```python
from build123d import *

# Parameters (mm, degrees)
F0_W     = 12.7
F0_H     = 21.59
F0_W_2   = 21.59
F0_H_2   = 12.7
F1_DEPTH = 50.8
F2_R     = 4.7625
F3_DEPTH = 12.7
F4_R     = 4.7625
F5_DEPTH = 12.7


with BuildPart() as f1:
    # F0 (on Top) → F1 (new body)
    with BuildSketch(Plane.XY):
        Polygon((34.29, 0), (0, 0), (0, -34.29), (12.7, -34.29), (12.7, -12.7), (34.29, -12.7), align=None)
        with Locations((6.35, -45.085)):
            Rectangle(F0_W, F0_H)
        with Locations((45.085, -6.35)):
            Rectangle(F0_W_2, F0_H_2)
    extrude(amount=F1_DEPTH)

    # F2 (on face) → F3 (join)
    with BuildSketch(Plane.XZ.offset(12.7)):
        with Locations((34.29, 25.4)):
            Circle(F2_R)
    extrude(amount=F3_DEPTH)

    # F4 (on face) → F5 (join)
    with BuildSketch(Plane.YZ.offset(12.7)):
        with Locations((-34.29, 25.4)):
            Circle(F4_R)
    extrude(amount=F5_DEPTH)


solid = f1.part
```
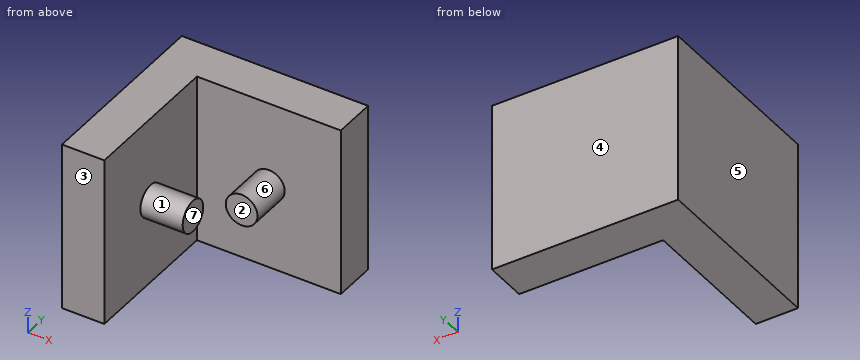
For this review, take the finished solid that the model builds, in its own axes (mm). Face numbers are marked on the shaded views. A direction names the side the tool comes from. Round coordinates to 2 decimals unless told otherwise and drop trailing zeros. Loops run counter-clockwise (first coordinate to the right, second up) from the corner with the lowest first, then second, coordinate; pieces in that order, holes last.
(1) We need section A-A (y = -21). Give the boundary of the cut face in (x, z) (1 decimal), plus the area to 3 significant figures.
Returned:
outline: (0, 0) - (12.7, 0) - (12.7, 50.8) - (0, 50.8) - close; circle Ø9.5 at (34.3, 25.4)
area: 716 mm2
(2) We need section D-D (x = 34.29). Give the boundary of the cut face in (y, z).
Returned:
outline: (-25.4, 20.64) - (-12.7, 20.64) - (-12.7, 0) - (0, 0) - (0, 50.8) - (-12.7, 50.8) - (-12.7, 30.16) - (-25.4, 30.16) - close
(3) We need section C-C (y = -34.29). Give the boundary of the cut face in (x, z), plus the area to 3 significant figures.
Returned:
outline: (0, 0) - (12.7, 0) - (12.7, 20.64) - (25.4, 20.64) - (25.4, 30.16) - (12.7, 30.16) - (12.7, 50.8) - (0, 50.8) - close
area: 766 mm2
(4) Wall thickness on line 1 along Y through (x, z) = (19, 41); line 2 along X through (y, z) = (-48, 5.5); line 3 along Y through (x, z) = (13, 24): over which ranges is each line inside the solid? List them lowest first.
Returned:
line 1: y = -12.7 to 0
line 2: x = 0 to 12.7
line 3: y = -38.84 to -29.74, -12.7 to 0
(5) Mouldability with a two-part tool opening along X and no side actions: class the marked faces 4, 5, 6 and 7 as released by +X, released by -X, zero draft, split by the parting line, or undercut.
Returned:
face 4: zero draft
face 5: released by -X
face 6: undercut
face 7: released by +X
(6) We need section B-B (z = 25.4). Give the boundary of the cut face in (x, y), plus the area to 3 significant figures.
Returned:
outline: (0, -55.88) - (12.7, -55.88) - (12.7, -39.05) - (25.4, -39.05) - (25.4, -29.53) - (12.7, -29.53) - (12.7, -12.7) - (29.53, -12.7) - (29.53, -25.4) - (39.05, -25.4) - (39.05, -12.7) - (55.88, -12.7) - (55.88, 0) - (0, 0) - close
area: 1,500 mm2
(7) Clearance check with flat-ended pins moving along their axes: P1, Ø21.5, axis at y = -24.5, z = 14.5, coming from the +X side; P2, Ø1, axis at x = 23.5, z = 7, coming from the -Y side; P3, Ø10, axis at x = 29.5, y = -39, coming from the +Z side. State where each tip first meets the part, or that it passes through.
Returned:
P1: stops at x = 39.05
P2: stops at y = -12.7
P3: stops at z = 29.79
(8) Tool access review of the marked faces 1, 2 and 3: name each direction out of +Z, -Z, +X, -X, +Y, -Y from which nothing blocks a thin tool from reaching the whole face with its end or side.
Returned:
face 1: +X
face 2: +Z, -Z, +X, -Y
face 3: +Z, -Z, +X, -X, -Y
